Autodesk Inventor part; units mm, degrees
ref_plane "YZ Plane" through (0, 0, 0) normal (1, 0, 0) x (0, 1, 0)
ref_plane "XZ Plane" through (0, 0, 0) normal (0, 1, 0) x (-1, 0, 0)
ref_plane "XY Plane" through (0, 0, 0) normal (0, 0, 1) x (1, 0, 0)
sketch "スケッチ1" plane through (0, 0, 0) normal (1, 0, 0) x (0, 1, 0)
  line L0 (-14.5, 81) -> (14.5, 81)
  line L1 (14.5, 81) -> (14.5, -81)
  line L2 (14.5, -81) -> (-14.5, -81)
  line L3 (-14.5, -81) -> (-14.5, 81)
  line L4 (-14.5, 81) -> (14.5, -81) construction
  line L5 (14.5, 81) -> (-14.5, -81) construction
  arc A0 (14.5, 55.8853) -> (0, 81) centre (-14.5, 55.8853) ccw
  arc A1 (0, 81) -> (-14.5, 55.8853) centre (14.5, 55.8853) ccw
  arc A2 (0, -81) -> (14.5, -55.8853) centre (-14.5, -55.8853) ccw
  arc A3 (-14.5, -55.8853) -> (0, -81) centre (14.5, -55.8853) ccw
  point P0 (0, 0)
  dimension "d0" = 29
  dimension "d1" = 162
extrude "押し出し1" add sketch "スケッチ1" along normal mid plane 126 contours A0 L1 A2 A3 L3 A1
fillet "フィレット1" radius 8 2 edges at (0, 0, 81) (0, 0, -81)
sketch "スケッチ2" plane through (63, 0, 0) normal (1, 0, 0) x (0, 0, -1)
  arc A0 (-76.8626, 5.5238) -> (-76.8626, -5.5238) centre (-71.0757, 0) ccw
  arc A1 (76.8626, -5.5238) -> (76.8626, 5.5238) centre (71.0757, 0) ccw
  line L0 (-71.0757, 0) -> (71.0757, 0) construction
  circle A2 centre (65.0757, 0) radius 3
  circle A3 centre (-16.9243, 0) radius 3
  line L1 (34.0757, 2.5) -> (47.0757, 2.5)
  line L2 (47.0757, 2.5) -> (47.0757, -2.5)
  line L3 (47.0757, -2.5) -> (34.0757, -2.5)
  line L4 (34.0757, -2.5) -> (34.0757, 2.5)
  line L5 (34.0757, 2.5) -> (47.0757, -2.5) construction
  line L6 (47.0757, 2.5) -> (34.0757, -2.5) construction
  line L7 (10.5757, 2.5) -> (23.5757, 2.5)
  line L8 (23.5757, 2.5) -> (23.5757, -2.5)
  line L9 (23.5757, -2.5) -> (10.5757, -2.5)
  line L10 (10.5757, -2.5) -> (10.5757, 2.5)
  line L11 (10.5757, 2.5) -> (23.5757, -2.5) construction
  line L12 (23.5757, 2.5) -> (10.5757, -2.5) construction
  line L13 (-4.9243, 0) -> (1.0757, 0) construction
  line L14 (-4.9243, -1.5) -> (1.0757, -1.5)
  line L15 (1.0757, 1.5) -> (-4.9243, 1.5)
  arc A4 (-4.9243, 1.5) -> (-4.9243, -1.5) centre (-4.9243, 0) ccw
  arc A5 (1.0757, -1.5) -> (1.0757, 1.5) centre (1.0757, 0) ccw
  point P0 (0, 0)
  point P1 (40.5757, 0)
  point P2 (17.0757, 0)
  point P3 (40.5757, 0)
  point P4 (17.0757, 0)
  point P5 (-1.9243, 0)
  point P6 (0, 0)
  dimension "d5" = 6
  dimension "d6" = 6
  dimension "d7" = 6
  dimension "d8" = 88
  dimension "d9" = 13
  dimension "d10" = 5
  dimension "d11" = 13
  dimension "d12" = 5
  dimension "d13" = 24.5
  dimension "d14" = 48
  dimension "d15" = 73
  dimension "d16" = 1.5
  dimension "d18" = 6
extrude "押し出し2" cut sketch "スケッチ2" against normal blind 5
properties part number "batter_krisdonia"
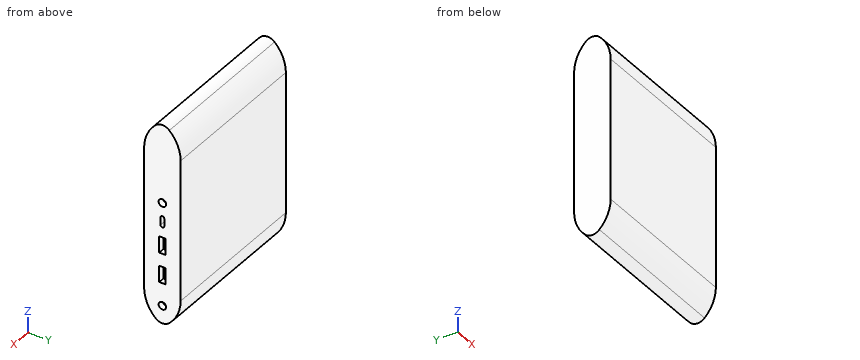
CAD build for the part. Positions are in the model's coordinates, mm. Round coordinates to 2 decimals unless told otherwise and drop trailing zeros. Order: outer loops, then holes, each group sorted by start corner. A loop starts at its lowest first (then second) coordinate and runs counter-clockwise, first axis right, second up.
Item 1: Saw through at A-A on z = -65. Write the cut outline in (x, y), then the cut area to 3 significant figures.
Item 2: Pin check, flat tips, straight feed: pin 1 (5 mm diameter, centred on x = 34, y = 6, fed in from +Z); pin 2 (3 mm diameter, centred on x = -42.5, y = -3.5, fed in from +Z); pin 3 (3 mm diameter, centred on y = -1, z = -66, fed in from +X). Stop position of each tip, or through.
Item 3: Probe line 1 along X through (y, z) = (-1.75, -47); line 2 along Y through (x, z) = (49, 57); line 3 along Z through (x, y) = (1, 2). List the from-to ranges inside material, lowest first.
Item 4: Saw through at B-B on y = -7.5. Write the cut outline in (x, z), then the cut area to 3 significant figures.
Reported:
1. outline: (-63, -13.03) - (63, -13.03) - (63, -3) - (58, -3) - (58, 3) - (63, 3) - (63, 13.03) - (-63, 13.03) - close
1. area: 3,250 mm2
2. pin 1: stops at z = 78.27
2. pin 2: stops at z = 78.82
2. pin 3: stops at x = 58
3. line 1: x = -63 to 58
3. line 2: y = -14.48 to 14.48
3. line 3: z = -78.82 to 78.82
4. outline: (-63, -74.78) - (63, -74.78) - (63, 74.78) - (-63, 74.78) - close
4. area: 18,800 mm2
